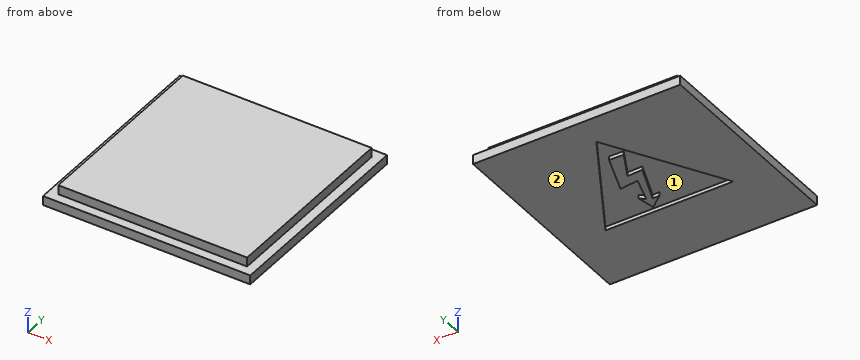
```python
from build123d import *

# Parameters (mm, degrees)
SKETCH2_W           = 56.2
SKETCH2_H           = 56.2
BOSS_EXTRUDE1_DEPTH = 2.5
SKETCH3_W           = 51.2
SKETCH3_H           = 51.2
BOSS_EXTRUDE2_DEPTH = 2.5
CUT_EXTRUDE1_DEPTH  = 1
BOSS_EXTRUDE3_DEPTH = 1


with BuildPart() as part:
    # Sketch2 → Boss-Extrude1 (new body)
    with BuildSketch(Plane.XY):
        Rectangle(SKETCH2_W, SKETCH2_H)
    extrude(amount=BOSS_EXTRUDE1_DEPTH)

    # Sketch3 → Boss-Extrude2 (add)
    with BuildSketch(Plane.XY.offset(2.5)):
        Rectangle(SKETCH3_W, SKETCH3_H)
    extrude(amount=BOSS_EXTRUDE2_DEPTH)

    # Sketch4 → Cut-Extrude1 (cut)
    with BuildSketch(Plane(origin=(0, 0, 0), x_dir=(-1, 0, 0), z_dir=(0, 0, -1))):
        Polygon((0, 20), (-17.320508076, -10), (17.320508076, -10), align=None)
    extrude(amount=-CUT_EXTRUDE1_DEPTH, mode=Mode.SUBTRACT)

    # Sketch5 → Boss-Extrude3 (add)
    with BuildSketch(Plane(origin=(0, 0, 1), x_dir=(-1, 0, 0), z_dir=(0, 0, -1))):
        Polygon((-1.517755642, 12.461495331), (-5.561610901, 1.642869574), (-0.574357926, 2.168045581), (-2.883213262, -4.921830522), (-4.196153281, -3.661408103), (-3.303354068, -8.387992172), (0.320360384, -5.447006529), (-1.517755642, -5.447006529), (2.631134818, 5.109031224), (-1.465238042, 4.951478422), (2.368546814, 12.356460129), align=None)
    extrude(amount=BOSS_EXTRUDE3_DEPTH)


solid = part.part
```
The model under review builds one solid part; all positions refer to its coordinate system, in mm. Face numbers are marked on the shaded views. Round coordinates to 2 decimals unless told otherwise and drop trailing zeros. Write each loop counter-clockwise with the first axis right and the second up, starting at its lowest first coordinate (ties: lowest second). Pieces come first, ordered by that corner, then holes.
(1) Wall thickness on L1, parallel to Y at x = -16.5, z = 2.8; L2, parallel to Z at x = 1.5, y = -8: over which ranges is each line inside the solid? List them lowest first.
(2) We need section B-B on x = -8. Give the boundary of the cut face in (y, z), and give its area (3 significant figures).
(3) Mouldability with a two-part tool opening along Y and no side actions: class the marked faces 1 and 2 as +Y half, -Y half, draft (parallel to the pull), parting line (faces both ways), or undercut.
(4) Insertion check: pin 1 (0.8 mm diameter, centred on y = 3.5, z = 4, fed in from -X); pin 2 (0.8 mm diameter, centred on x = -6, z = 4, fed in from +Y); pin 3 (1.2 mm diameter, centred on x = 11.5, z = 4, fed in from -Y). Each pin has a flat end and moves straight along its axis. Give the tip position at first contact, or say it passes through.
(5) We need section A-A on y = -23. Give the boundary of the cut face in (x, z).
(6) We need section D-D on y = -6.5. Give the boundary of the cut face in (x, z).
(7) We need section C-C on z = 4.25. Give the boundary of the cut face in (x, y), and give its area (3 significant figures).
Findings below:
1. L1: y = -25.6 to 25.6
1. L2: z = 1 to 5
2. outline: (-28.1, 0) - (-10, 0) - (-10, 1) - (6.14, 1) - (6.14, 0) - (28.1, 0) - (28.1, 2.5) - (25.6, 2.5) - (25.6, 5) - (-25.6, 5) - (-25.6, 2.5) - (-28.1, 2.5) - close
2. area: 252 mm2
3. face 1: undercut
3. face 2: draft
4. pin 1: stops at x = -25.6
4. pin 2: stops at y = 25.6
4. pin 3: stops at y = -25.6
5. outline: (-28.1, 0) - (28.1, 0) - (28.1, 2.5) - (25.6, 2.5) - (25.6, 5) - (-25.6, 5) - (-25.6, 2.5) - (-28.1, 2.5) - close
6. outline: (-28.1, 0) - (-15.3, 0) - (-15.3, 1) - (0.98, 1) - (0.98, 0) - (3.66, 0) - (3.66, 1) - (15.3, 1) - (15.3, 0) - (28.1, 0) - (28.1, 2.5) - (25.6, 2.5) - (25.6, 5) - (-25.6, 5) - (-25.6, 2.5) - (-28.1, 2.5) - close
7. outline: (-25.6, -25.6) - (25.6, -25.6) - (25.6, 25.6) - (-25.6, 25.6) - close
7. area: 2,620 mm2
